from build123d import *

# Parameters (mm, degrees)
SKETCH1_W           = 38.1
SKETCH1_H           = 38.1
BOSS_EXTRUDE1_DEPTH = 7.62
SKETCH2_W           = 25.4
SKETCH2_H           = 25.4
BOSS_EXTRUDE2_DEPTH = 19.05
CUT_EXTRUDE1_REACH  = 9.62
SKETCH3_R           = 3.81
CUT_EXTRUDE2_DEPTH  = 6.35
CUT_EXTRUDE3_REACH  = 40.1


with BuildPart() as part:
    # Sketch1 → Boss-Extrude1 (new body)
    with BuildSketch(Plane(origin=(0, 0, 0), x_dir=(1, 0, 0), z_dir=(0, 1, 0))):
        Rectangle(SKETCH1_W, SKETCH1_H)
    extrude(amount=BOSS_EXTRUDE1_DEPTH)

    # Sketch2 → Boss-Extrude2 (add)
    with BuildSketch(Plane(origin=(0, 7.62, 0), x_dir=(1, 0, 0), z_dir=(0, 1, 0))):
        with Locations((-6.35, 6.35)):
            Rectangle(SKETCH2_W, SKETCH2_H)
    extrude(amount=BOSS_EXTRUDE2_DEPTH)

    # Sketch3 → Cut-Extrude1 (cut, up to next)
    with BuildSketch(Plane(origin=(0, 7.62, 0), x_dir=(1, 0, 0), z_dir=(0, 1, 0)), mode=Mode.PRIVATE) as cut_extrude1_sk1:
        with Locations((12.7, 12.7)):
            Circle(SKETCH3_R)
    cut_extrude1_tool1 = extrude(cut_extrude1_sk1.sketch, amount=-CUT_EXTRUDE1_REACH, mode=Mode.PRIVATE) & part.part
    add(cut_extrude1_tool1.solids().sort_by_distance((12.7, 7.62, -12.7))[0], mode=Mode.SUBTRACT)
    # Sketch3 → Cut-Extrude1 (cut, up to next)
    with BuildSketch(Plane(origin=(0, 7.62, 0), x_dir=(1, 0, 0), z_dir=(0, 1, 0)), mode=Mode.PRIVATE) as cut_extrude1_sk2:
        with Locations((-12.7, -12.7)):
            Circle(SKETCH3_R)
    cut_extrude1_tool2 = extrude(cut_extrude1_sk2.sketch, amount=-CUT_EXTRUDE1_REACH, mode=Mode.PRIVATE) & part.part
    add(cut_extrude1_tool2.solids().sort_by_distance((-12.7, 7.62, 12.7))[0], mode=Mode.SUBTRACT)

    # Sketch4 → Cut-Extrude2 (cut)
    with BuildSketch(Plane.ZY.offset(19.05)):
        Polygon((-13.335, 21.59), (-10.541, 21.59), (-10.541, 10.414), (0.635, 10.414), (0.635, 7.62), (-13.335, 7.62), align=None)
    extrude(amount=-CUT_EXTRUDE2_DEPTH, mode=Mode.SUBTRACT)

    # Sketch5 → Cut-Extrude3 (cut, up to next)
    with BuildSketch(Plane.ZY.offset(19.05), mode=Mode.PRIVATE) as cut_extrude3_sk1:
        Polygon((-6.35, 26.67), (6.35, 7.62), (6.35, 26.67), align=None)
    cut_extrude3_tool1 = extrude(cut_extrude3_sk1.sketch, amount=-CUT_EXTRUDE3_REACH, mode=Mode.PRIVATE) & part.part
    add(cut_extrude3_tool1.solids().sort_by_distance((-19.05, 20.32, 2.116667))[0], mode=Mode.SUBTRACT)


solid = part.part
Can you work these out from the model? Positions are in its coordinate system, mm. A direction names the side the tool comes from. Give positions to 0.01 mm unless a question says otherwise; leave off trailing zeros. Loops run counter-clockwise (first coordinate to the right, second up) from the corner with the lowest first, then second, coordinate; pieces in that order, holes last. Notation, with made-up numbers: (-31.75, 44.25) - (-12.75, 44.25) arc R25 ccw to (-12.75, 72.25) - close; hole circle Ø6 at (36, 47). An arc over 180 degrees is marked (long way). Return JSON: item names as keys, results as strings.
1. If I drill on line 1 (Z direction, x = 12.7, y = 5.75); line 2 (Z direction, x = -12.7, y = 3.75), over which ranges is the centre line in solid material (lowest first)?
Output values:
{"line 1": "z = -19.05 to -16.51, -8.89 to 19.05", "line 2": "z = -19.05 to 8.89, 16.51 to 19.05"}
2. I want a section at B-B on z = -12.7. Please give me the cut outline in (x, y).
Output values:
{"outline": "(-19.05, 0) - (8.89, 0) - (8.89, 7.62) - (6.35, 7.62) - (6.35, 26.67) - (-19.05, 26.67) - (-19.05, 21.59) - (-12.7, 21.59) - (-12.7, 7.62) - (-19.05, 7.62) - close; (16.51, 0) - (19.05, 0) - (19.05, 7.62) - (16.51, 7.62) - close"}
3. I want a section at A-A on x = 12.7. Please give me the cut outline in (y, z).
Output values:
{"outline": "(0, -19.05) - (7.62, -19.05) - (7.62, -16.51) - (0, -16.51) - close; (0, -8.89) - (7.62, -8.89) - (7.62, 19.05) - (0, 19.05) - close"}
4. For faces 4 (the face through (-16, 10.414, -5)), 5 (the face through (8, 7.62, 4)), 6 (the face through (6.35, 17, -9)), which set-ups out of +Z, -Z, +X, -X, +Y, -Y let a thin tool reach every point of the face, with its end or its side?
Output values:
{"face 4": "-X", "face 5": "+Z, +X, +Y", "face 6": "+Z, -Z, +X, +Y"}
5. I'm going to push flat-ended pins straight in: pin 1 Ø5.5 at (y, z) = (17, -3) entering from +X; pin 2 Ø6 at (y, z) = (23, 2.5) entering from -X; pin 3 Ø9 at (x, z) = (-12.7, 12.7) entering from +Y; pin 4 Ø1.5 at (x, y) = (-10.5, 11) entering from +Z. Where does each tip first touch, or does it pass through?
Output values:
{"pin 1": "stops at x = 6.35", "pin 2": "passes through", "pin 3": "stops at y = 7.62", "pin 4": "stops at z = 4.6"}
6. I want a section at D-D on x = -15. Please give me the cut outline in (y, z) (3 decimals).
Output values:
{"outline": "(0, -19.05) - (26.67, -19.05) - (26.67, -6.35) - (7.62, 6.35) - (7.62, 9.663) - (0, 9.663) - close; (0, 15.737) - (7.62, 15.737) - (7.62, 19.05) - (0, 19.05) - close; hole (7.62, -13.335) - (21.59, -13.335) - (21.59, -10.541) - (10.414, -10.541) - (10.414, 0.635) - (7.62, 0.635) - close"}
7. We'd pull the mould along Z, two halves only. Please class faces 1 (the face through (-16, 9, 0.635)), 2 (the face through (0, 4, 19.05)), 3 (the face through (-7, 26.67, -13)): +Z half, -Z half, draft (parallel to the pull), parting line (faces both ways), or undercut.
Output values:
{"face 1": "undercut", "face 2": "+Z half", "face 3": "draft"}
8. I want a section at C-C on y = 3. Please give me the cut outline in (x, z), and give its area (3 significant figures).
Output values:
{"outline": "(-19.05, -19.05) - (19.05, -19.05) - (19.05, 19.05) - (-19.05, 19.05) - close; hole circle Ø7.62 at (-12.7, 12.7); hole circle Ø7.62 at (12.7, -12.7)", "area": "1,360 mm²"}
